```python
from build123d import *

# Parameters (mm, degrees)
F0_W     = 15.24
F0_H     = 15.24
F0_H_2   = 274.32
F1_DEPTH = 203.2
F2_W     = 299.72
F2_H     = 304.8
F3_DEPTH = 15.24
F4_W     = 299.72
F4_H     = 355.6
F5_DEPTH = 12.7
F6_W     = 76.2
F6_H     = 152.4
F7_DEPTH = 25.4
F9_DEPTH = 373.126


with BuildPart() as f1:
    # F0 (on Top) → F1 (new body)
    with BuildSketch(Plane.XY):
        Polygon((-33.02, 137.16), (-33.02, 152.4), (-149.86, 152.4), (-149.86, -152.4), (-33.02, -152.4), (-33.02, -137.16), (-134.62, -137.16), (-134.62, 137.16), align=None)
        with Locations((-25.4, 144.78)):
            Rectangle(F0_W, F0_H)
        with Locations((-25.4, -144.78)):
            Rectangle(F0_W, F0_H)
        with Locations((-25.4, 0)):
            Rectangle(F0_W, F0_H_2)
        Polygon((149.86, -152.4), (149.86, 152.4), (-17.78, 152.4), (-17.78, 137.16), (134.62, 137.16), (134.62, -137.16), (-17.78, -137.16), (-17.78, -152.4), align=None)
    extrude(amount=F1_DEPTH)

    # F2 (on face) → F3 (join)
    with BuildSketch(Plane(origin=(0, 0, 0), x_dir=(1, 0, 0), z_dir=(0, 0, -1))):
        Rectangle(F2_W, F2_H)
    extrude(amount=F3_DEPTH)

    # F4 (on face) → F5 (join)
    with BuildSketch(Plane.XY.offset(203.2)):
        Rectangle(F4_W, F4_H)
    extrude(amount=F5_DEPTH)

    # F6 (on face) → F7 (cut)
    with BuildSketch(Plane(origin=(0, 152.4, 0), x_dir=(-1, 0, 0), z_dir=(0, 1, 0))):
        with Locations((83.82, 76.2)):
            Rectangle(F6_W, F6_H)
    extrude(amount=-F7_DEPTH, mode=Mode.SUBTRACT)

    # F8 (on face) → F9 (cut)
    with BuildSketch(Plane.YZ.offset(149.86)):
        Polygon((-177.8, 207.01), (177.8, 215.9), (-177.8, 215.9), align=None)
    extrude(amount=-F9_DEPTH, mode=Mode.SUBTRACT)


solid = f1.part
```
Source: CAD feature listing. Evaluate the final solid. Frame: model axes, mm. A direction names the side the tool comes from. Coordinates: 2 decimals unless noted, no trailing zeros. Loops run counter-clockwise (first coordinate to the right, second up) from the corner with the lowest first, then second, coordinate; pieces in that order, holes last. Notation, with made-up numbers: M 37,-36.75 L 70,-36.75 A10 cw 70,-18.75 Z; hole C 48.25,17 d7. An arc over 180 degrees is marked long. Use a Markdown table: item, result. Add a question column.
Q1. Draft query along Y for faces 6 (the flat face through (-2, 177.8, 209)), 7 (the flat face through (-83, 10, 0)), 8 (the flat face through (-45.72, 145, 75)). Return one class per face: pulls with the +Y half, pulls with the -Y half, needs draft (parallel to the pull), parting line crosses it, or undercut.
Q2. Section query D-D, the plane z = 96.5. Return loops of the section in (x, y).
Q3. Access query for faces 1 (the flat face through (-149.86, -2, 99)), 2 (the flat face through (57, 2, 203.2)), 3 (the flat face through (-2, -165, 203.2)), 4 (the flat face through (-83, 145, 152.4)), 5 (the flat face through (-2, 165, 203.2)). Directions: +Z, -Z, +X, -X, +Y, -Y. A direction counts if a zero-diameter tool reaches every point of the face in a straight line with its end or side. Return the directions, or none.
Q4. Section query B-B, the plane z = 169. Return loops of the section in (x, y), and give its area (3 significant figures).
Q5. Material intervals for L1, parallel to X at y = -69.5, z = 175.5; L2, parallel to Y at x = 5.5, z = 51; L3, parallel to Y at x = -31.5, z = 153, sorted ascending.
Q6. Section query C-C, the plane y = 25. Return loops of the section in (x, z).
Q7. Section query A-A, the plane x = 111. Return loops of the section in (y, z), and give its area (3 significant figures).
Q8. First-contact query: pin 1 (4 mm diameter, centred on x = 111, z = 174.5, fed in from -Y); pin 2 (7.5 mm diameter, centred on x = -40, y = -160.5, fed in from -Z); pin 3 (1 mm diameter, centred on x = 88, z = 75, fed in from +Y). Flat tips, straight axial feed; report the tip coordinate or a pass-through.
Result:
| question | item | result |
|---|---|---|
| 1 | face 6 | pulls with the +Y half |
| 1 | face 7 | undercut |
| 1 | face 8 | needs draft |
| 2 | outline | M -149.86,-152.4 L 149.86,-152.4 L 149.86,152.4 L -45.72,152.4 L -45.72,137.16 L -33.02,137.16 L -33.02,-137.16 L -134.62,-137.16 L -134.62,137.16 L -121.92,137.16 L -121.92,152.4 L -149.86,152.4 Z; hole M -17.78,-137.16 L 134.62,-137.16 L 134.62,137.16 L -17.78,137.16 Z |
| 3 | face 1 | +Z, -Z, -X, +Y, -Y |
| 3 | face 2 | none |
| 3 | face 3 | -Z, +X, -X, -Y |
| 3 | face 4 | +Y |
| 3 | face 5 | -Z, +X, -X, +Y |
| 4 | outline | M -149.86,-152.4 L 149.86,-152.4 L 149.86,152.4 L -149.86,152.4 Z; hole M -134.62,-137.16 L -33.02,-137.16 L -33.02,137.16 L -134.62,137.16 Z; hole M -17.78,-137.16 L 134.62,-137.16 L 134.62,137.16 L -17.78,137.16 Z |
| 4 | area | 21,700 mm2 |
| 5 | L1 | x = -149.86 to -134.62, -33.02 to -17.78, 134.62 to 149.86 |
| 5 | L2 | y = -152.4 to -137.16, 137.16 to 152.4 |
| 5 | L3 | y = -152.4 to 152.4 |
| 6 | outline | M -149.86,-15.24 L 149.86,-15.24 L 149.86,212.08 L -149.86,212.08 Z; hole M -134.62,0 L -33.02,0 L -33.02,203.2 L -134.62,203.2 Z; hole M -17.78,0 L 134.62,0 L 134.62,203.2 L -17.78,203.2 Z |
| 7 | outline | M -177.8,203.2 L -152.4,203.2 L -152.4,-15.24 L 152.4,-15.24 L 152.4,203.2 L 177.8,203.2 L 177.8,215.9 L -177.8,207.01 Z; hole M -137.16,0 L 137.16,0 L 137.16,203.2 L -137.16,203.2 Z |
| 7 | area | 13,800 mm2 |
| 8 | pin 1 | stops at y = -152.4 |
| 8 | pin 2 | stops at z = 203.2 |
| 8 | pin 3 | stops at y = 152.4 |
